Geometry check sheet. Reference: drawing and pictorial views, mm from the part's lowest x, y, z. Coordinates: 2 decimals unless noted, no trailing zeros. Loops run counter-clockwise (first coordinate to the right, second up) from the corner with the lowest first, then second, coordinate; pieces in that order, holes last. Notation, with made-up numbers: (-29.5, 6.5) - (-24.5, 6.5) arc R18 ccw to (-24.5, 17.5) - close; hole circle Ø8 at (80, -5). An arc over 180 degrees is marked (long way). One line per item, written item: value.
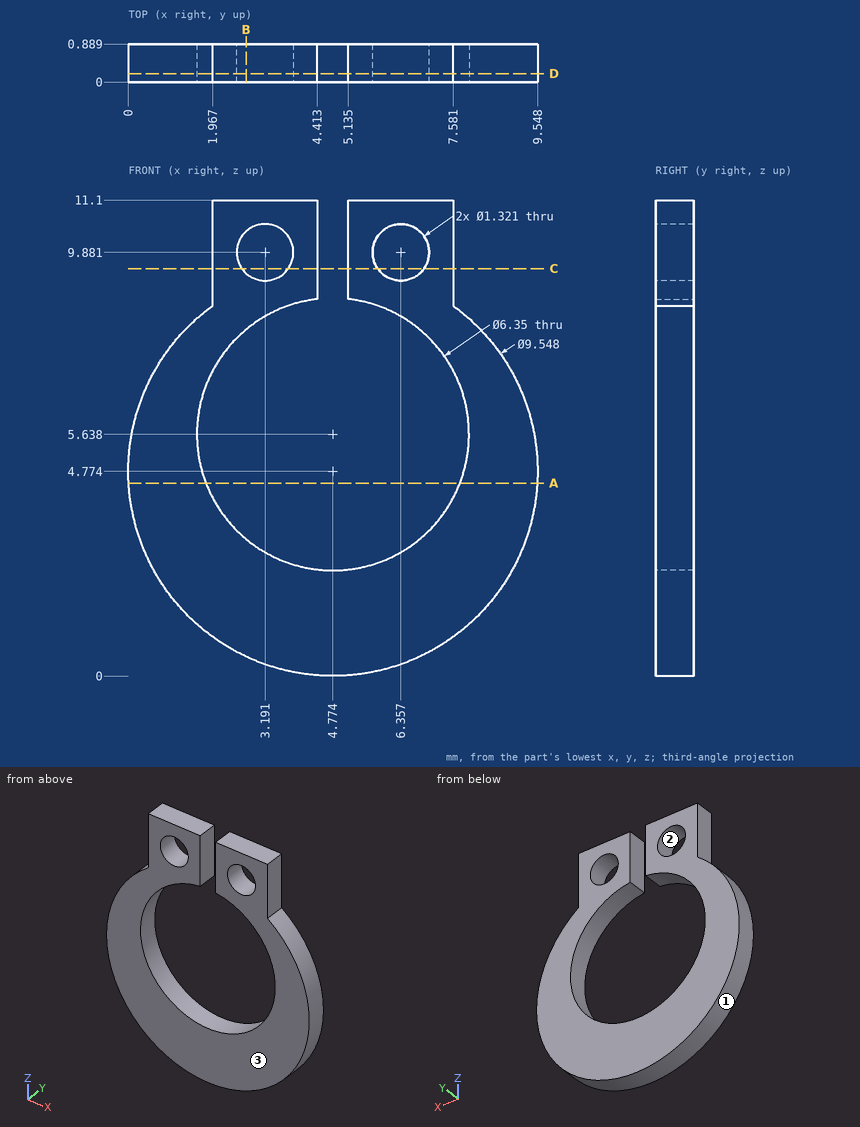
(1) Cross-section at C-C on z = 9.5. Record the cut outline in (x, y) (1 decimal).
Reply:
outline: (2, 0) - (2.7, 0) - (2.7, 0.9) - (2, 0.9) - close; (3.7, 0) - (4.4, 0) - (4.4, 0.9) - (3.7, 0.9) - close; (5.1, 0) - (5.8, 0) - (5.8, 0.9) - (5.1, 0.9) - close; (6.9, 0) - (7.6, 0) - (7.6, 0.9) - (6.9, 0.9) - close
(2) Go/stop test with a flat-tipped pin: pin 1 Ø4 at (x, z) = (4.77, 5.64) entering from +Y. Record where the tip stops, or that it passes through.
Reply:
pin 1: through
(3) Release check for a two-part mould opening along Z. For the marked faces 1, 2 and 3 record: pulls with the +Z half, pulls with the -Z half, needs draft (parallel to the pull), parting line crosses it, or undercut.
Reply:
face 1: parting line crosses it
face 2: undercut
face 3: needs draft
(4) Cross-section at D-D on y = 0.2. State how many separate pieces and enclosed holes the cut face has.
Reply:
separate pieces: 1
enclosed holes: 2
(5) Cross-section at A-A on z = 4.5. Record the cut outline in (x, y).
Reply:
outline: (0.01, 0) - (1.81, 0) - (1.81, 0.89) - (0.01, 0.89) - close; (7.74, 0) - (9.54, 0) - (9.54, 0.89) - (7.74, 0.89) - close
(6) Cross-section at B-B on x = 2.75. Record the cut outline in (y, z).
Reply:
outline: (0, 0.45) - (0.89, 0.45) - (0.89, 3.19) - (0, 3.19) - close; (0, 8.08) - (0.89, 8.08) - (0.89, 9.39) - (0, 9.39) - close; (0, 10.37) - (0.89, 10.37) - (0.89, 11.1) - (0, 11.1) - close
(7) Material ranges on probe 1 along Z at (x, y) = (3.25, 0.8); probe 2 along Z at (x, y) = (6, 0.6) (1 decimal); probe 3 along Z at (x, y) = (5.5, 0.2) (1 decimal), recorded low to high. Write a range as from..to.
Reply:
probe 1: 0.25..2.85, 8.42..9.22, 10.54..11.1
probe 2: 0.2..2.7, 8.6..9.3, 10.4..11.1
probe 3: 0.1..2.5, 8.7..11.1
